Part model, mm, in its own coordinate system. A direction names the side the tool comes from. Round coordinates to 2 decimals unless told otherwise and drop trailing zeros. Write each loop counter-clockwise with the first axis right and the second up, starting at its lowest first coordinate (ties: lowest second). Pieces come first, ordered by that corner, then holes.
Autodesk Inventor part; units mm, degrees
ref_plane "YZ Plane" through (0, 0, 0) normal (1, 0, 0) x (0, 1, 0)
ref_plane "XZ Plane" through (0, 0, 0) normal (0, 1, 0) x (-1, 0, 0)
ref_plane "XY Plane" through (0, 0, 0) normal (0, 0, 1) x (1, 0, 0)
sketch "sk_main" plane through (0, 0, 0) normal (1, 0, 0) x (0, 1, 0)
  line L0 (-10, 0) -> (42.5, 0)
  line L1 (0, -15.4) -> (0, 15.4)
  line L2 (25, -9) -> (0, -9)
  line L3 (0, -9) -> (0, 9)
  line L4 (0, 9) -> (25, 9)
  line L5 (25, 9) -> (25, -9)
  line L6 (25, -9) -> (0, 9) construction
  line L7 (0, -9) -> (25, 9) construction
  circle A0 centre (30, 0) radius 1.75
  circle A1 centre (30, 0) radius 5 construction
  line L8 (-2.5, 11) -> (31, 11)
  line L9 (31, 11) -> (31, 4.899)
  line L10 (31, -4.899) -> (31, -11)
  line L11 (31, -11) -> (-2.5, -11)
  line L12 (-2.5, -11) -> (-2.5, 11)
  arc A2 (31, -4.899) -> (31, 4.899) centre (30, 0) ccw
  line L13 (0, 11) -> (0, -11)
  point P0 (0, 0)
  point P1 (12.5, 0)
  dimension "d0" = 25
  dimension "d1" = 18
  dimension "d2" = 3.5
  dimension "d3" = 5
  dimension "d4" = 2
  dimension "d5" = 2.5
  dimension "d6" = 1
extrude "ext_main_back" add sketch "sk_main" along normal mid plane 6 contours L5 L4 L1 L8 L9 A2 L0 A0 | L0 A0 A2 L10 L11 L1 L2 L5
extrude "ext_main_front" add sketch "sk_main" along normal mid plane 12.15 contours L12 L8 L1 L0 | L0 L1 L11 L12
sketch "sk_front" plane through (0, 0, 0) normal (0, 1, 0) x (-1, 0, 0)
  line L0 (0, -15.4) -> (0, 15.4)
  line L1 (8.505, 0) -> (-8.505, 0)
  circle A0 centre (0, 0) radius 3.4
  circle A1 centre (5.075, 0) radius 1
  circle A2 centre (-5.075, 0) radius 1
  circle A3 centre (0, 0) radius 8 construction
  circle A4 centre (0, -9) radius 8 construction
  circle A5 centre (0, -9) radius 1
  circle A6 centre (8.6494, -4.5) radius 1.75 construction
  circle A7 centre (-8.6494, -4.5) radius 1.75 construction
  line L2 (8.6494, -4.5) -> (-8.6494, -4.5) construction
  line L3 (-6.075, 11) -> (-6.075, -11)
  line L4 (6.075, -11) -> (6.075, 11)
  line L5 (10.3994, 1) -> (10.3994, -7)
  line L6 (10.3994, 1) -> (6.075, 11)
  line L7 (10.3994, -7) -> (6.075, -11)
  line L8 (-6.075, 11) -> (-10.3994, 1)
  line L9 (-10.3994, 1) -> (-10.3994, -7)
  line L10 (-10.3994, -7) -> (-6.075, -11)
  line L11 (6.075, -11) -> (-6.075, -11)
  circle A8 centre (-8.6494, -4.5) radius 1
  circle A9 centre (8.6494, -4.5) radius 1
  circle A10 centre (-5, 8.5) radius 1
  circle A11 centre (-5, 8.5) radius 2.25 construction
  line L12 (-5, 8.5) -> (5, 8.5) construction
  circle A12 centre (5, 8.5) radius 2.25 construction
  circle A13 centre (5, 8.5) radius 1
  point P0 (0, 8.5)
  dimension "d11" = 6.8
  dimension "d12" = 2
  dimension "d13" = 10.15
  dimension "d14" = 16
  dimension "d15" = 16
  dimension "d16" = 9
  dimension "d17" = 2
  dimension "d18" = 3.5
  dimension "d21" = 8
  dimension "d22" = 4
  dimension "d26" = 2
  dimension "d27" = 2
  dimension "d28" = 4.5
  dimension "d30" = 10
  dimension "d31" = 8.5
extrude "ext_front_tabs" add sketch "sk_front" against normal up to surface (2.5 mm away) contours L4 L6 L5 L7 | L10 L9 L8 L3 | A8 | A9
extrude "ext_cut_holesfront" cut sketch "sk_front" against normal through all contours A5 L0 | L0 A5 | A1 L1 | L1 A1 | A2 L1 | L1 A2 | A0 L1 L0 | L0 L1 A0 | L1 A0 L0 | L0 A0 L1 | A8 | A9 | A10 | A13
fillet "Fillet2" radius 2 2 edges at (3, 0, 10) (-3, 0, 10)
fillet "Fillet3" radius 3 2 edges at (3, 0, -10) (-3, 0, -10)
fillet "Fillet4" radius 4 2 edges at (0, 31, 11) (0, 31, -11)
extrude "ext_dowelfill" add sketch "sk_front" against normal blind 1.65 contours A5 L0 | L0 A5
equation "\"d2\" = screw_m3_bore_loose"
equation "\"d12\" = screw_m2_bore_selfthreading"
equation "\"d17\" = screw_m2_bore_selfthreading"
equation "\"d26\" = screw_m2_bore_selfthreading"
equation "\"d27\" = screw_m2_bore_selfthreading"
equation "\"d28\" = screw_m2_head_maxsize"
properties part number "empty"
Q1. Drop flat-ended pins along their axis: pin 1 (5 mm diameter, centred on x = 7, y = 30.5, fed in from -Z); pin 2 (6 mm diameter, centred on y = 15, z = 7.5, fed in from +X); pin 3 (0.6 mm diameter, centred on x = 0.5, z = 6, fed in from +Y); pin 4 (0.6 mm diameter, centred on x = 0, z = -9.5, fed in from -Y). Give the stop position or say it passes through.
Values follow:
pin 1: passes through
pin 2: stops at x = 3
pin 3: stops at y = 31
pin 4: stops at y = -1.65
Q2. Which spindle directions (+Z, -Z, +X, -X, +Y, -Y) get a long thin tool onto all of the face, cutting with end or side? Do faces 5 (the cylindrical face through (0.042, 29.797, -9.859)), 6 (the flat face through (0, 31, 6)), 7 (the flat face through (0, 13, -9)), 8 (the cylindrical face through (3.6, 0.57, 9.99)), 9 (the cylindrical face through (9.386, -1.232, -3.824)). Say none if no direction does.
Values follow:
face 5: -Z, +X, -X, +Y
face 6: +Z, +X, -X, +Y
face 7: +X, -X
face 8: +Z, +X, +Y
face 9: +Y, -Y
Q3. Cut at C-C on y = 1. Write the cut outline in (x, z), plus the area to 3 significant figures.
Values follow:
outline: (-3.76, -11) - (3.76, -11) - (3.76, -9) - (-3.76, -9) - close; (-3.27, 9) - (3.27, 9) - (3.27, 11) - (-3.27, 11) - close
area: 28.1 mm2
Q4. Mould opens along X. For faces 1 (the flat face through (3, 26, 0)), 2 (the cylindrical face through (0, 35, 0)), 3 (the cylindrical face through (6.074, -1.232, 0.044)), 4 (the cylindrical face through (-3.57, 0.6, 9.99)) say: +X half, -X half, draft (parallel to the pull), parting line (faces both ways), or undercut.
Values follow:
face 1: +X half
face 2: draft
face 3: undercut
face 4: -X half
Q5. Cut at D-D on y = 26.5. Write the cut outline in (x, z).
Values follow:
outline: (-3, -11) - (3, -11) - (3, 11) - (-3, 11) - close
Q6. Cut at A-A on z = -0.5. Write the cut outline in (x, y).
Values follow:
outline: (-10.4, -2.5) - (-5.94, -2.5) - (-5.94, 0) - (-10.4, 0) - close; (-4.21, -2.5) - (-3.36, -2.5) - (-3.36, 0) - (-4.21, 0) - close; (-3, 25) - (3, 25) - (3, 28.32) - (-3, 28.32) - close; (-3, 31.68) - (3, 31.68) - (3, 34.97) - (-3, 34.97) - close; (3.36, -2.5) - (4.21, -2.5) - (4.21, 0) - (3.36, 0) - close; (5.94, -2.5) - (10.4, -2.5) - (10.4, 0) - (5.94, 0) - close
Q7. Cut at B-B on x = 0. Write the cut outline in (y, z).
Values follow:
outline: (-2.5, -11) - (27, -11) arc R4 ccw to (31, -7) - (31, -4.9) arc R5 ccw to (31, 4.9) - (31, 7) arc R4 ccw to (27, 11) - (-2.5, 11) - (-2.5, 3.4) - (0, 3.4) - (0, 9) - (25, 9) - (25, -9) - (0, -9) - (0, -3.4) - (-2.5, -3.4) - (-2.5, -8) - (-1.65, -8) - (-1.65, -10) - (-2.5, -10) - close; hole circle Ø3.5 at (30, 0)
Q8. Wall check: L1, parallel to X at y = -0.95, z = 0 (3 decimals); L2, parallel to Z at x = 5, y = -1.65; L3, parallel to Y at x = 2.25, z = -5.75. Give the ranges that are in metal, low to high.
Values follow:
L1: x = -10.399 to -6.075, -4.075 to -3.4, 3.4 to 4.075, 6.075 to 10.399
L2: z = -11 to -1, 1 to 7.5, 9.5 to 11
L3: y = -2.5 to 0, 25 to 31
